from build123d import *

# Parameters (mm, degrees)
BOSS_EXTRU_1_DEPTH     = 36
CHANFREIN1_SIZE        = 11.24
CHANFREIN1_EDGE_2_SIZE = 11.24
CHANFREIN1_EDGE_3_SIZE = 11.24
CHANFREIN2_SIZE        = 2
CHANFREIN3_SIZE        = 2


with BuildPart() as part:
    # Esquisse1 → Boss.-Extru.1 (new body)
    with BuildSketch(Plane(origin=(0, 0, 0), x_dir=(1, 0, 0), z_dir=(0, 1, 0))):
        Polygon((-70, 0), (70, 0), (0, 121.24355653), align=None)
    extrude(amount=BOSS_EXTRU_1_DEPTH)

    # Chanfrein1
    chanfrein1_edges = [part.edges().sort_by_distance(p)[0] for p in [
        (70, 18, 0),
    ]]
    chamfer(chanfrein1_edges, length=CHANFREIN1_SIZE)

    # Chanfrein1 edge 2
    chanfrein1_edge_2_edges = [part.edges().sort_by_distance(p)[0] for p in [
        (-70, 18, 0),
    ]]
    chamfer(chanfrein1_edge_2_edges, length=CHANFREIN1_EDGE_2_SIZE)

    # Chanfrein1 edge 3
    chanfrein1_edge_3_edges = [part.edges().sort_by_distance(p)[0] for p in [
        (0, 18, -121.24355653),
    ]]
    chamfer(chanfrein1_edge_3_edges, length=CHANFREIN1_EDGE_3_SIZE)

    # Chanfrein2
    chanfrein2_edges = [part.edges().sort_by_distance(p)[0] for p in [
        (0, 36, 0),
        (-35, 36, -60.621778265),
        (35, 36, -60.621778265),
        (61.57, 36, -4.867062769),
        (0, 36, -111.509430991),
        (-61.57, 36, -4.867062769),
    ]]
    chamfer(chanfrein2_edges, length=CHANFREIN2_SIZE)

    # Chanfrein3
    chanfrein3_edges = [part.edges().sort_by_distance(p)[0] for p in [
        (0, 0, 0),
        (35, 0, -60.621778265),
        (-35, 0, -60.621778265),
        (61.57, 0, -4.867062769),
        (0, 0, -111.509430991),
        (-61.57, 0, -4.867062769),
    ]]
    chamfer(chanfrein3_edges, length=CHANFREIN3_SIZE)


solid = part.part
Read the model definition and answer for the solid it produces. Units are mm, in the model's axes. Round coordinates to 2 decimals unless told otherwise and drop trailing zeros. Loops run counter-clockwise (first coordinate to the right, second up) from the corner with the lowest first, then second, coordinate; pieces in that order, holes last.
Q1. Section A-A on z = -41.5 is taken. Write down the section's boundary in (x, y).
Q2. Section C-C on y = 11.5 is taken. Write down the section's boundary in (x, z).
Q3. Section B-B on x = -43.5 is taken. Write down the section's boundary in (y, z), and give its area (3 significant figures).
Q4. Each of these flat-tipped pins is pushed along its axis until it touches: pin 1 (12 mm diameter, centred on y = 14, z = -69, fed in from +X); pin 2 (12 mm diameter, centred on y = 16, z = -31, fed in from -X). Where does it stop, or does it pass through?
Q5. Consider probe 1 along Z at (x, y) = (21, 7); probe 2 along X at (y, z) = (5.5, -15.5); probe 3 along X at (y, z) = (34.5, -101). Determine where each line is inside the solid, lowest interval first.
Output:
1. outline: (-46.04, 2) - (-43.73, 0) - (43.73, 0) - (46.04, 2) - (46.04, 34) - (43.73, 36) - (-43.73, 36) - (-46.04, 34) - close
2. outline: (-64.38, -9.73) - (-5.62, -111.51) - (5.62, -111.51) - (64.38, -9.73) - (58.76, 0) - (-58.76, 0) - close
3. outline: (0, -41.9) - (2, -45.9) - (34, -45.9) - (36, -41.9) - (36, -2) - (34, 0) - (2, 0) - (0, -2) - close
3. area: 1,640 mm2
4. pin 1: stops at x = 33.63
4. pin 2: stops at x = -55.57
5. probe 1: z = -84.87 to 0
5. probe 2: x = -61.05 to 61.05
5. probe 3: x = -11.11 to 11.11
